from build123d import *

# Parameters (mm, degrees)
BOSS_EXTRUDE1_DEPTH = 6
SKETCH3_R           = 2
CUT_EXTRUDE1_DEPTH  = 55.481648286
SKETCH4_R           = 2
CUT_EXTRUDE2_DEPTH  = 52.886896226
FILLET1_R           = 3
FILLET2_R           = 1


with BuildPart() as part:
    # Sketch2 → Boss-Extrude1 (new body)
    with BuildSketch(Plane(origin=(0, 0, 0), x_dir=(1, 0, 0), z_dir=(0, 1, 0))):
        Polygon((-21, 17.5), (-21, -47.5), (-15, -47.5), (-15, -37.5), (-12, -17.5), (-1, -37.5), (-1, -47.5), (5, -47.5), (5, -37.5), (-15, 17.5), (-15, 27.5), (-21, 27.5), align=None)
    extrude(amount=BOSS_EXTRUDE1_DEPTH)

    # Sketch3 → Cut-Extrude1 (cut, through all)
    with BuildSketch(Plane(origin=(5, 0, 0), x_dir=(0, 0, -1), z_dir=(1, 0, 0))):
        with Locations((-42.5, 3)):
            Circle(SKETCH3_R)
    extrude(amount=-CUT_EXTRUDE1_DEPTH, mode=Mode.SUBTRACT)

    # Sketch4 → Cut-Extrude2 (cut, through all)
    with BuildSketch(Plane(origin=(-15, 0, 0), x_dir=(0, 0, -1), z_dir=(1, 0, 0))):
        with Locations((22.5, 3)):
            Circle(SKETCH4_R)
    extrude(amount=-CUT_EXTRUDE2_DEPTH, mode=Mode.SUBTRACT)

    # Fillet1
    fillet1_edges = [part.edges().sort_by_distance(p)[0] for p in [
        (-18, 0, -27.5),
        (-18, 6, -27.5),
        (2, 0, 47.5),
        (2, 6, 47.5),
        (-18, 0, 47.5),
        (-18, 6, 47.5),
    ]]
    fillet(fillet1_edges, radius=FILLET1_R - 0.0001)  # a hair under: the kernel refuses the full size

    # Fillet2
    fillet2_edges = [part.edges().sort_by_distance(p)[0] for p in [
        (-15, 0, -21.00005),
        (-5, 0, 10),
        (-1, 0, 41.00005),
        (-6.5, 0, 27.5),
        (-13.5, 0, 27.5),
        (-13.5, 6, 27.5),
        (-12, 3, 17.5),
        (-15, 3, 37.5),
        (-6.5, 6, 27.5),
        (-1, 6, 41.00005),
        (-5, 6, 10),
        (-15, 6, -21.00005),
        (-21, 0, 10),
        (-21, 6, 10),
        (-21, 5.121349633, 46.621349633),
        (-21, 0.878650367, 46.621349633),
        (-21, 5.121349633, -26.621349633),
        (-21, 0.878650367, -26.621349633),
        (5, 0, 41.00005),
        (-15, 0, 41.00005),
        (-15, 5.121349633, -26.621349633),
        (-15, 0.878650367, -26.621349633),
        (-15, 6, 41.00005),
        (5, 6, 41.00005),
        (5, 5.121349633, 46.621349633),
        (5, 0.878650367, 46.621349633),
        (-1, 5.121349633, 46.621349633),
        (-1, 0.878650367, 46.621349633),
        (-15, 5.121349633, 46.621349633),
        (-15, 0.878650367, 46.621349633),
    ]]
    fillet(fillet2_edges, radius=FILLET2_R - 0.0001)  # a hair under: the kernel refuses the full size


solid = part.part
The model under review builds one solid part; all positions refer to its coordinate system, in mm. A direction names the side the tool comes from. Round coordinates to 2 decimals unless told otherwise and drop trailing zeros. One line per question, with ' | ' between items. Start each with the question number.
Item 1: For pin 1 (2 mm diameter, centred on x = -7, y = 2, fed in from +Z); pin 2 (1.5 mm diameter, centred on x = -15.5, y = 4.5, fed in from -Z); pin 3 (2 mm diameter, centred on y = 5.5, z = -16.5, fed in from +X), all flat-tipped, find the tip position at first contact; note any pin that passes through.
Item 2: Wall thickness on line 1 along Y through (x, z) = (-18.35, -22.5); line 2 along X through (y, z) = (5.75, 37); line 3 along X through (y, z) = (1, 27.5): over which ranges is each line inside the solid? List them lowest first. Write a range as [from, to].
Item 3: Add section A-A, the plane z = 42.5. Count the separate pieces of the cut face and the enclosed holes in it, then the cut area to 3 significant figures.
Item 4: Machinability: for faces 1 (the face through (-13.732, 2.972, 29.045)), 2 (the face through (5, 3, 40)), 3 (the face through (-13.99, 0.29, 28.76)), 4 (the face through (-13.99, 5.71, 28.76)), 5 (the face through (-15, 3, -20)), which of the approach directions +Z, -Z, +X, -X, +Y, -Y give a long, thin tool a straight path to every point of the face, cutting with its end or side? Answer none if there is none.
Item 5: Draft analysis for pull direction Y (two halves, no side actions). For faces 6 (the face through (2.03, 0.86, 46.6)), 7 (the face through (-5, 3, 10)), 8 (the face through (2.042, 3.088, 44.498)), state which applies: +Y half, -Y half, draft (parallel to the pull), parting line (faces both ways), or undercut.
Return value:
1) pin 1: stops at z = 28.41 | pin 2: stops at z = -27.37 | pin 3: stops at x = -14.31
2) line 1: y = [0, 1], [5, 6] | line 2: x = [-20.66, -15.27], [-0.89, 4.46] | line 3: x = [-21, -13.5], [-6.5, 1.36]
3) separate pieces: 4 | enclosed holes: 0 | area: 22.3 mm2
4) face 1: +Z, +Y, -Y | face 2: +Z, -Z, +X, +Y, -Y | face 3: +Z, -Y | face 4: +Z, +Y | face 5: -Z, +X, +Y, -Y
5) face 6: -Y half | face 7: draft | face 8: undercut
